Work out the finished part from the listing and answer in its coordinate system (mm). A direction names the side the tool comes from. Round coordinates to 2 decimals unless told otherwise and drop trailing zeros. Write each loop counter-clockwise with the first axis right and the second up, starting at its lowest first coordinate (ties: lowest second). Pieces come first, ordered by that corner, then holes. Notation, with made-up numbers: (30.5, 25) - (70.5, 25) arc R14 cw to (70.5, 34) - close; hole circle Ø3 at (39, 46). An arc over 180 degrees is marked (long way). Answer as a JSON object with one key per item and string values.
Autodesk Inventor part; units mm, degrees
ref_plane "Arbeitsebene1" through (0, 0, 10) normal (0, 0, 1) x (1, 0, 0)
ref_plane "Arbeitsebene3" through (0, 0, 50) normal (0, 0, 1) x (1, 0, 0)
ref_plane "Arbeitsebene4" through (0, 0, 130) normal (0, 0, 1) x (1, 0, 0)
sketch "Skizze1" plane through (0, 0, 0) normal (0, 0, 1) x (1, 0, 0)
  circle A0 centre (0, 0) radius 30
  circle A1 centre (0, 0) radius 13.5
  circle A2 centre (0, 0) radius 9.5
  circle A3 centre (0, 0) radius 23.25 construction
  line L0 (0, 0) -> (0, 23.25) construction
  point P0 (-23.25, 0)
  point P1 (0, -23.25)
  point P2 (23.25, 0)
  dimension "d4" = 46.5
  dimension "d0" = 4
  dimension "d1" = 27
  dimension "d3" = 30
  dimension "d7" = 360
extrude "Extrusion1" add sketch "Skizze1" along normal blind 10 contours A0 | A1
extrude "Extrusion2" add sketch "Skizze1" against normal blind 2.6 contours A1
sketch "Skizze2" plane through (0, 0, 10) normal (0, 0, 1) x (1, 0, 0)
  point P0 (0, 0)
  point P1 (0, 23.25)
  point P2 (20.1351, 11.625)
  point P3 (20.1351, -11.625)
  point P4 (23.25, 0)
  point P5 (0, -23.25)
  point P6 (-23.25, 0)
hole "Bohrung1" at (0, 23.25, 10) at (20.1351, 11.625, 10) at (20.1351, -11.625, 10) at (23.25, 0, 10) at (0, -23.25, 10) at (-23.25, 0, 10) direction (0, 0, -1) diameter 4.134 end through all
ref_plane "Arbeitsebene1" through (0, 0, 10) normal (0, 0, 1) x (1, 0, 0)
sketch "Skizze4" plane through (0, 0, 0) normal (1, 0, 0) x (0, 1, 0)
  line L0 (9.5, -2.6) -> (-9.5, -2.6) construction
  line L1 (0, 192.52) -> (0, -35.12) construction
  line L2 (-9.5, 10) -> (-9.5, -2.6) construction
  line L3 (9.5, 10) -> (9.5, -2.6) construction
  line L4 (-9.5, 10) -> (9.5, 10) construction
  line L5 (-9.5, 2.4) -> (9.5, 2.4)
  line L6 (-9.5, 2.4) -> (-9.5, 10)
  line L7 (-9.5, 10) -> (-20, 10)
  line L8 (-20, 10) -> (-20, 160)
  line L9 (-20, 160) -> (20, 160)
  line L10 (20, 10) -> (9.5, 10)
  line L11 (9.5, 10) -> (9.5, 2.4)
  line L12 (20, 160) -> (20, 10)
  line L13 (0, 2.4) -> (0, 160)
  point P0 (0, 0)
  dimension "d27" = 5
  dimension "d31" = 150
  dimension "d33" = 40
revolve "Umdrehung1" add sketch "Skizze4" angle 360 about axis through (0, 0, 0) along (0, 0, -1) contours L13 L9 L12 L10 L11 L5
sketch "Skizze5" plane through (0, 0, 160) normal (0, 0, 1) x (1, 0, 0)
  circle A0 centre (0, 0) radius 20
  line L0 (-12, 16) -> (-12, -16)
  line L1 (12, 16) -> (12, -16)
  line L2 (-6.245, 19) -> (6.245, 19)
  circle A1 centre (0, 0) radius 20 construction
  dimension "MainAxis_Schluesselweite" = 24
  dimension "d46" = 1
  dimension "d52" = 32
extrude "Extrusion3" cut sketch "Skizze5" against normal blind 140 contours A0 L1 | A0 L0
sketch "Skizze6" plane through (0, 0, 0) normal (1, 0, 0) x (0, 1, 0)
  line L0 (-16, 160) -> (16, 160) construction
  line L1 (-16, 20) -> (16, 20) construction
  line L2 (0, -32) -> (0, 192) construction
  line L3 (-16, 20) -> (-16, 160)
  line L4 (16, 160) -> (16, 20)
  point P0 (0, 0)
  dimension "Flansch_ParralelMech_FlatPart_Width" = 140
ref_plane "Arbeitsebene2" through (0, 0, 90) normal (0, 0, 1) x (1, 0, 0)
ref_plane "Arbeitsebene3" through (0, 0, 50) normal (0, 0, 1) x (1, 0, 0)
ref_plane "Arbeitsebene4" through (0, 0, 130) normal (0, 0, 1) x (1, 0, 0)
extrude "Extrusion4" cut sketch "Skizze5" against normal blind 140 contours L2 A0
sketch "Skizze7" plane through (0, 0, 50) normal (0, 0, 1) x (1, 0, 0)
  line L0 (-12, 16) -> (-12, -16) construction
  line L1 (-12, 15) -> (-3, 15)
  line L2 (-3, 15) -> (-3, 11.425)
  line L3 (-3, 11.425) -> (3, 11.425)
  line L4 (3, 11.425) -> (3, 15)
  line L5 (3, 15) -> (12, 15)
  line L6 (-12, 0) -> (-12, 15)
  line L7 (0, -16) -> (0, 16) construction
  line L8 (12, -16) -> (12, 16) construction
  line L9 (12, 15) -> (12, 0)
  line L10 (-12, 0) -> (12, 0)
  line L11 (-42, 0) -> (42, 0) construction
  point P0 (0, 11.425)
  point P1 (-12, -7.2111)
  point P2 (12, 7.2111)
  dimension "d51" = 9
  dimension "d63" = 30
  dimension "d64" = 22.85
revolve "Umdrehung2" cut sketch "Skizze7" angle 360 about axis through (-10, 0, 50) along (1, 0, 0)
ref_plane "Arbeitsebene5" through (0, 0, 85) normal (1, 0, 0) x (0, 0, -1)
sketch "Skizze8" plane through (12, -16, 160) normal (1, 0, 0) x (0, 0, -1)
  line L0 (30, -26) -> (30, 58) construction
  line L1 (-32.52, 16) -> (195.12, 16) construction
  point P0 (160, 16)
  point P1 (30, 16)
hole "Bohrung2" at (12, 0, 130) direction (-1, 0, 0) diameter 6.647 end through all
mirror "Spiegeln2" about plane through (0, 0, 0) normal (0, 1, 0) of "Extrusion4"
equation "\"d4\" = Flansch_FemalePart_HoleDia"
equation "\"d1\" = Flansch_Klemmdeckelausnahme_Dia"
equation "\"d3\" = Flansch_FemalePart_OuterDia"
equation "\"d47\" = Flansch_ParralelMech_FlatPart_Width"
equation "\"d33\" = d28"
equation "\"Total_Bearing_Hole_Dist\" = 80"
properties part number "Flansch_FemalePart_MainAxis_HeadConnectorBase" material "Edelstahl"
Item 1: A cutting plane is placed at A-A (x = 0). Give the number of separate pieces and of enclosed holes in the cut face, and give its area (3 significant figures).
Results found:
{"separate pieces": "3", "enclosed holes": "2", "area": "5,770 mm²"}
Item 2: A cutting plane is placed at D-D (z = 95.5). Write down the section's boundary in (x, y) (3 decimals).
Results found:
{"outline": "(-12, -16) arc R20 ccw to (-6.245, -19) - (6.245, -19) arc R20 ccw to (12, -16) - (12, 16) arc R20 ccw to (6.245, 19) - (-6.245, 19) arc R20 ccw to (-12, 16) - close"}
Item 3: Consider line 1 along Y through (x, z) = (0, 0.5); line 2 along Z through (x, y) = (6.25, 0); line 3 along Y through (x, z) = (-4.25, 130). Determine where each line is inside the solid, lowest interval first.
Results found:
{"line 1": "-30 to -25.32, -21.18 to -9.5, 9.5 to 21.18, 25.32 to 30", "line 2": "2.4 to 35, 65 to 126.68, 133.32 to 160", "line 3": "-19 to -3.32, 3.32 to 19"}
Item 4: Determine the mould class of faces 1 (the cylindrical face through (0.042, 6.142, 59.634)), 2 (the flat face through (12, 0, 107)), 3 (the cylindrical face through (-25, -1.1, 4.9)) for opening direction X: pulls with the +X half, pulls with the -X half, needs draft (parallel to the pull), parting line crosses it, or undercut.
Results found:
{"face 1": "needs draft", "face 2": "pulls with the +X half", "face 3": "undercut"}
Item 5: A cutting plane is placed at B-B (z = 50). Write down the section's boundary in (x, y) (3 decimals), and give its area (3 significant figures).
Results found:
{"outline": "(-12, -16) arc R20 ccw to (-6.245, -19) - (6.245, -19) arc R20 ccw to (12, -16) - (12, -15) - (3, -15) - (3, -11.425) - (-3, -11.425) - (-3, -15) - (-12, -15) - close; (-12, 15) - (-3, 15) - (-3, 11.425) - (3, 11.425) - (3, 15) - (12, 15) - (12, 16) arc R20 ccw to (6.245, 19) - (-6.245, 19) arc R20 ccw to (-12, 16) - close", "area": "205 mm²"}
Item 6: For faces 4 (the flat face through (-3, 4, 39)), 5 (the flat face through (0, 19, 91)), 6 (the flat face through (0, 0, 2.4)), 7 (the flat face through (-12, 0, 107)), 8 (the flat face through (-20.4, 0.4, 10)), determine the directions among +Z, -Z, +X, -X, +Y, -Y from which every point of the face is accessible in a straight line to the end or side of a thin tool.
Results found:
{"face 4": "-X", "face 5": "+Z, +X, -X, +Y", "face 6": "-Z", "face 7": "+Z, -X, +Y, -Y", "face 8": "+Z"}
Item 7: Each of these flat-tipped pins is pushed along its axis until it touches: P1, Ø8, axis at y = 1, z = 102.5, coming from the +X side; P2, Ø5, axis at x = 0, y = -23.25, coming from the +Z side; P3, Ø3.5, axis at x = 1, z = 62.5, coming from the +Y side; P4, Ø2, axis at y = -21.5, z = 97, coming from the -X side. Where does it stop, or does it pass through?
Results found:
{"P1": "x = 12", "P2": "z = 10", "P3": "y = 19", "P4": "through"}
